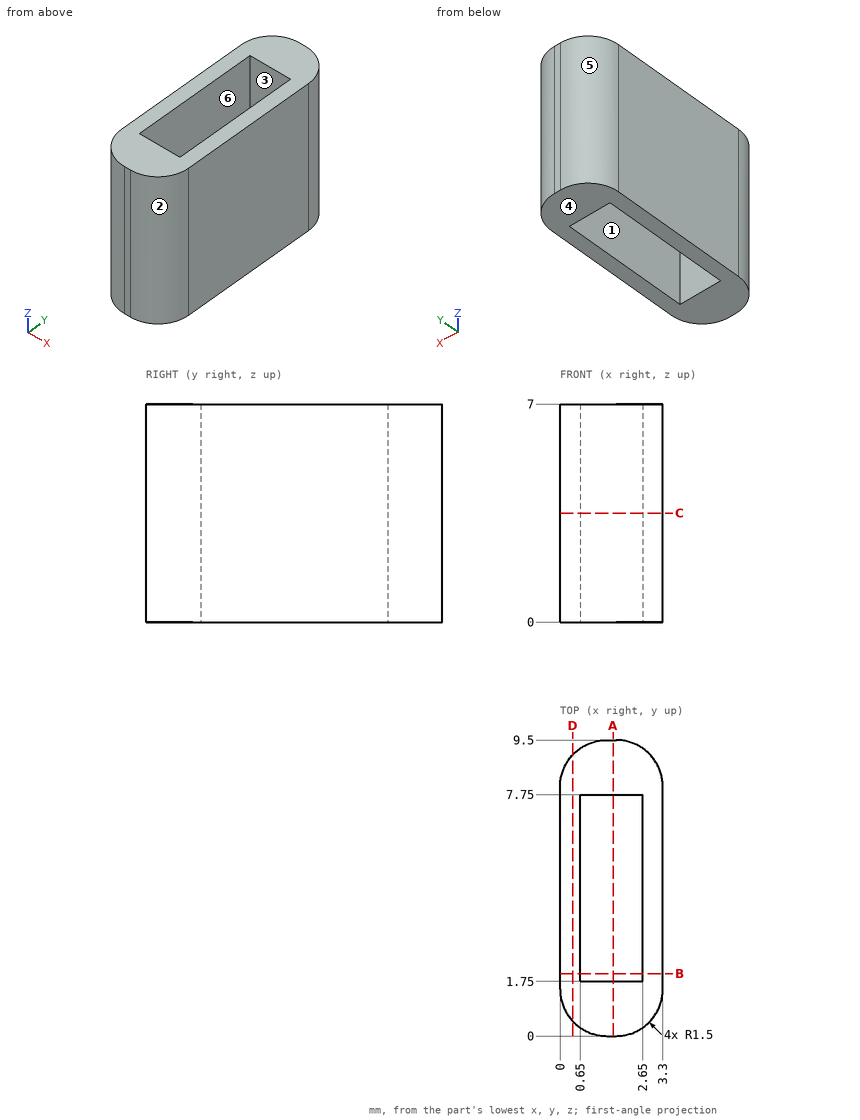
Answer from the drawing. Dimensions are ordinates in mm from the lowest x, y and z of the part. A direction names the side the tool comes from. Coordinates: 2 decimals unless noted, no trailing zeros. Order: outer loops, then holes, each group sorted by start corner. A loop starts at its lowest first (then second) coordinate and runs counter-clockwise, first axis right, second up. Notation, with made-up numbers: M -25,86.5 L -19,86.5 A25 cw -19,107.5 Z; hole C 57,51.25 d4. An arc over 180 degrees is marked long. Put each result on its own line as item: value. Start each with the question number.
Item 1: For the marked faces 5 and 6, determine the directions among +Z, -Z, +X, -X, +Y, -Y from which every point of the face is accessible in a straight line to the end or side of a thin tool.
Item 2: Section C-C, the plane z = 3.5 is taken. Determine the outline of the cut face in (x, y), plus the area to 3 significant figures.
Item 3: The mould has two halves that part along X. Classify the marked faces 1, 2, 3 and 4: +X half, -X half, draft (parallel to the pull), parting line (faces both ways), or undercut.
Item 4: Section D-D, the plane x = 0.4 is taken. Determine the outline of the cut face in (y, z), plus the area to 3 significant figures.
Item 5: Section A-A, the plane x = 1.7 is taken. Determine the outline of the cut face in (y, z), plus the area to 3 significant figures.
Item 6: Section B-B, the plane y = 2 is taken. Determine the outline of the cut face in (x, z).
Item 7: Consider probe 1 along X at (y, z) = (3.25, 6.5); probe 2 along Y at (x, z) = (1.75, 1.5); probe 3 along Y at (x, z) = (2.55, 2.5). Determine where each line is inside the solid, lowest interval first. Write a range as [from, to].
Computed:
1. face 5: +Z, -Z, -X, +Y
1. face 6: +Z, -Z
2. outline: M 0,1.5 A1.5 ccw 1.5,0 L 1.8,0 A1.5 ccw 3.3,1.5 L 3.3,8 A1.5 ccw 1.8,9.5 L 1.5,9.5 A1.5 ccw 0,8 Z; hole M 0.65,1.75 L 2.65,1.75 L 2.65,7.75 L 0.65,7.75 Z
2. area: 17.4 mm2
3. face 1: undercut
3. face 2: +X half
3. face 3: undercut
3. face 4: draft
4. outline: M 0.48,0 L 9.02,0 L 9.02,7 L 0.48,7 Z
4. area: 59.8 mm2
5. outline: M 0,0 L 1.75,0 L 1.75,7 L 0,7 Z; M 7.75,0 L 9.5,0 L 9.5,7 L 7.75,7 Z
5. area: 24.5 mm2
6. outline: M 0,0 L 0.65,0 L 0.65,7 L 0,7 Z; M 2.65,0 L 3.3,0 L 3.3,7 L 2.65,7 Z
7. probe 1: x = [0, 0.65], [2.65, 3.3]
7. probe 2: y = [0, 1.75], [7.75, 9.5]
7. probe 3: y = [0.2, 1.75], [7.75, 9.3]
